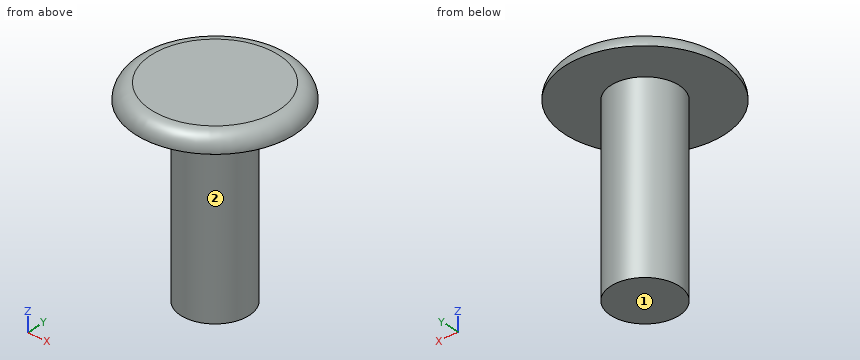
Autodesk Inventor part; units mm, degrees
ref_plane "YZ Plane" through (0, 0, 0) normal (1, 0, 0) x (0, 1, 0)
ref_plane "XZ Plane" through (0, 0, 0) normal (0, 1, 0) x (-1, 0, 0)
ref_plane "XY Plane" through (0, 0, 0) normal (0, 0, 1) x (1, 0, 0)
sketch "スケッチ1" plane through (0, 0, 0) normal (0, 0, 1) x (1, 0, 0)
  circle A0 centre (0, 0) radius 3.5
  dimension "d0" = 7
extrude "押し出し1" add sketch "スケッチ1" along normal blind 0.7
sketch "スケッチ2" plane through (0, 0, 0) normal (0, 0, -1) x (-1, 0, 0)
  circle A0 centre (0, 0) radius 1.5
  dimension "d3" = 3
extrude "押し出し2" add sketch "スケッチ2" along normal blind 8
thread "ねじ1"
fillet "フィレット1" radius 0.7 1 edges at (-3.5, 0, 0.7)
properties part number "ネジ低頭m3.08" material "鋼、高強度、低合金"
Here's how the part is built. I have some questions about the finished solid (model axes, mm). Face numbers are marked on the shaded views. A direction names the side the tool comes from. Coordinates: 2 decimals unless noted, no trailing zeros. Order: outer loops, then holes, each group sorted by start corner. A loop starts at its lowest first (then second) coordinate and runs counter-clockwise, first axis right, second up. Notation, with made-up numbers: (-28.5, -13) -> (25.5, -13) arc R16 ccw to (25.5, 8) -> close; hole circle Ø7 at (-19.75, 61.25). An arc over 180 degrees is marked (long way). Return JSON: item names as keys, results as strings.
1) On a 3-axis mill with a long thin cutter (end or side, diameter ignored), from which of +Z, -Z, +X, -X, +Y, -Y can I reach the whole of each face in a straight line? I mean the marked faces 1 and 2. Say none if no direction works.
Conclusion:
{"face 1": "-Z, +X, -X, +Y, -Y", "face 2": "-Z"}
2) I'm going to push flat-ended pins straight in: P1, Ø3, axis at y = -1.5, z = -2, coming from the +X side; P2, Ø4, axis at y = -0.5, z = -1, coming from the +X side; P3, Ø1.5, axis at x = 2.5, y = 1, coming from the -Z side; P4, Ø2, axis at x = 2, z = -2.5, coming from the +Y side. Where does each tip first touch, or does it pass through?
Conclusion:
{"P1": "stops at x = 1.5", "P2": "stops at x = 3.5", "P3": "stops at z = 0", "P4": "stops at y = 1.12"}
3) If I drill on probe 1 along Z at (x, y) = (2, -2); probe 2 along Y at (x, z) = (0, -4.5); probe 3 along Y at (x, z) = (-3, 0.25), over which ranges is the centre line in solid material (lowest first)?
Conclusion:
{"probe 1": "z = 0 to 0.7", "probe 2": "y = -1.5 to 1.5", "probe 3": "y = -1.71 to 1.71"}
4) If we section it at C-C on z = -4: List the corners of the cut face in (x, y) for me.
Conclusion:
{"outline": "circle Ø3 at (0, 0)"}
